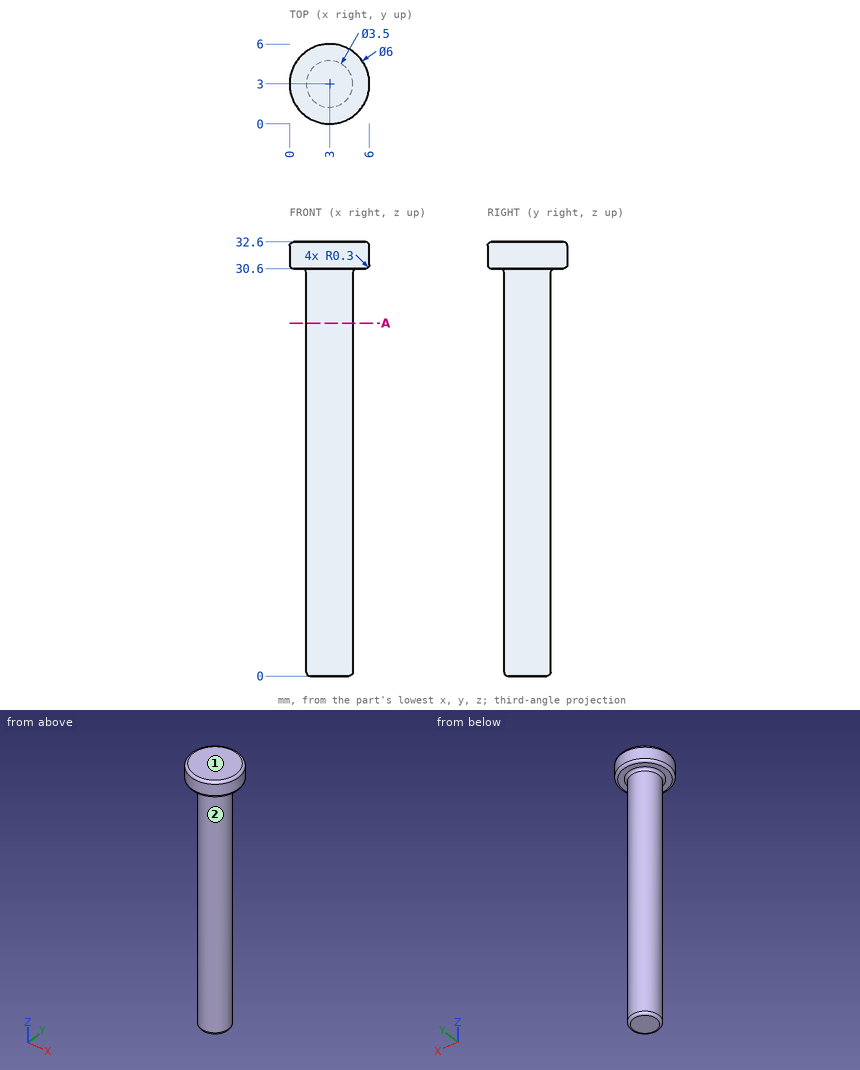
Here's the drawing with two shaded views (mm, measured from the low corner). I have some questions. Give positions to 0.01 mm unless a question says otherwise; leave off trailing zeros. Loops run counter-clockwise (first coordinate to the right, second up) from the corner with the lowest first, then second, coordinate; pieces in that order, holes last. Notation, with made-up numbers: (43, 68.5) -> (67, 68.5) arc R32 cw to (67, 106.5) -> close; hole circle Ø1 at (42, -37). An arc over 180 degrees is marked (long way). One line per item, written item: value.
Q1. Suppose I cut it at A-A on z = 26.5. Please give me the cut outline in (x, y), then the cut area to 3 significant figures.
Answers follow:
outline: circle Ø3.5 at (3, 3)
area: 9.62 mm^2
Q2. If I drill on line 1 along Z through (x, y) = (5.25, 1.5); line 2 along Y through (x, z) = (1.5, 17.5); line 3 along Y through (x, z) = (4, 5), over which ranges is the centre line in solid material (lowest first)?
Answers follow:
line 1: 30.6 to 32.6
line 2: 2.1 to 3.9
line 3: 1.56 to 4.44
Q3. We'd pull the mould along Y, two halves only. Please class the marked faces 1 and 2: pulls with the +Y half, pulls with the -Y half, needs draft (parallel to the pull), parting line crosses it, or undercut.
Answers follow:
face 1: needs draft
face 2: parting line crosses it
Q4. I'm going to push flat-ended pins straight in: pin 1 Ø2 at (x, z) = (4.5, 23) entering from +Y; pin 2 Ø1.5 at (x, z) = (1.5, 11.5) entering from +Y; pin 3 Ø1.5 at (x, z) = (4, 3.5) entering from -Y. Where does each tip first touch, or does it pass through?
Answers follow:
pin 1: y = 4.68
pin 2: y = 4.58
pin 3: y = 1.27
